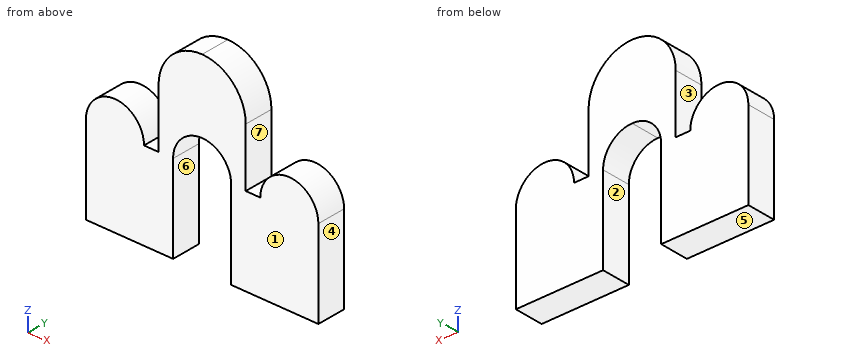
from build123d import *

# Parameters (mm, degrees)
F1_DEPTH = 10


with BuildPart() as f1:
    # F0 (on Front) → F1 (new body)
    with BuildSketch(Plane.XZ):
        with BuildLine():
            Line((0, 30), (0, 0))
            Line((0, 0), (30, 0))
            Line((30, 0), (30, 30))
            ThreePointArc((30, 30), (32.928932, 37.071068), (40, 40))
            ThreePointArc((40, 40), (47.071068, 37.071068), (50, 30))
            Line((50, 30), (50, 0))
            Line((50, 0), (80, 0))
            Line((80, 0), (80, 30))
            ThreePointArc((80, 30), (70, 40), (60, 30))
            Line((60, 30), (55, 30))
            Line((55, 30), (55, 50))
            ThreePointArc((55, 50), (50.606602, 60.606602), (40, 65))
            ThreePointArc((40, 65), (29.393398, 60.606602), (25, 50))
            Line((25, 50), (25, 30))
            Line((25, 30), (20, 30))
            ThreePointArc((20, 30), (10, 40), (0, 30))
        make_face()
    extrude(amount=F1_DEPTH)


solid = f1.part
Source: CAD feature listing. Evaluate the final solid. Frame: model axes, mm. Face numbers are marked on the shaded views. A direction names the side the tool comes from. Coordinates: 2 decimals unless noted, no trailing zeros. Order: outer loops, then holes, each group sorted by start corner. A loop starts at its lowest first (then second) coordinate and runs counter-clockwise, first axis right, second up.
Item 1: First-contact query: P1, Ø2, axis at x = 30, y = -8, coming from the +Z side; P2, Ø5, axis at y = -3, z = 41.5, coming from the +X side; P3, Ø4, axis at y = -5, z = 49.5, coming from the -X side; P4, Ø6, axis at x = 33, z = 51, coming from the +Y side. Flat tips, straight axial feed; report the tip coordinate or a pass-through.
Output values:
P1: stops at z = 62
P2: stops at x = 74.36
P3: stops at x = 25
P4: stops at y = 0
Item 2: Pull-direction query (X, two-part tool) for the marked faces 1, 2, 3 and 4; classes: pulls with the +X half, pulls with the -X half, needs draft (parallel to the pull), parting line crosses it, or undercut.
Output values:
face 1: needs draft
face 2: undercut
face 3: undercut
face 4: pulls with the +X half
Item 3: Cut plane B-B (z = 31.5). Return loops of the section in (x, y), plus the area to 3 significant figures.
Output values:
outline: (0.11, -10) - (19.89, -10) - (19.89, 0) - (0.11, 0) - close; (25, -10) - (30.11, -10) - (30.11, 0) - (25, 0) - close; (49.89, -10) - (55, -10) - (55, 0) - (49.89, 0) - close; (60.11, -10) - (79.89, -10) - (79.89, 0) - (60.11, 0) - close
area: 498 mm2
Item 4: Cut plane D-D (z = 47). Return loops of the section in (x, y), plus the area to 3 significant figures.
Output values:
outline: (25, -10) - (55, -10) - (55, 0) - (25, 0) - close
area: 300 mm2
Item 5: Set-up query: the marked faces 5, 6 and 7. Return all of +Z, -Z, +X, -X, +Y, -Y with unobstructed straight access to the full face (end or side cutting, diameter ignored); none if empty.
Output values:
face 5: -Z, +X, -X, +Y, -Y
face 6: -Z, +Y, -Y
face 7: +Z, +Y, -Y
Item 6: Cut plane C-C (x = 70). Return loops of the section in (y, z).
Output values:
outline: (-10, 0) - (0, 0) - (0, 40) - (-10, 40) - close
Item 7: Material intervals for line 1 (X direction, y = -0.5, z = 16.5); line 2 (X direction, y = -8.5, z = 31.5); line 3 (Z direction, x = 23, y = -9), sorted ascending.
Output values:
line 1: x = 0 to 30, 50 to 80
line 2: x = 0.11 to 19.89, 25 to 30.11, 49.89 to 55, 60.11 to 79.89
line 3: z = 0 to 30
Item 8: Cut plane A-A (z = 21.5). Return loops of the section in (x, y).
Output values:
outline: (0, -10) - (30, -10) - (30, 0) - (0, 0) - close; (50, -10) - (80, -10) - (80, 0) - (50, 0) - close
